Source: three-view drawing plus pictorial views. Frame: mm from the lowest corner of the part. Give positions to 0.01 mm unless a question says otherwise; leave off trailing zeros. Loops run counter-clockwise (first coordinate to the right, second up) from the corner with the lowest first, then second, coordinate; pieces in that order, holes last.
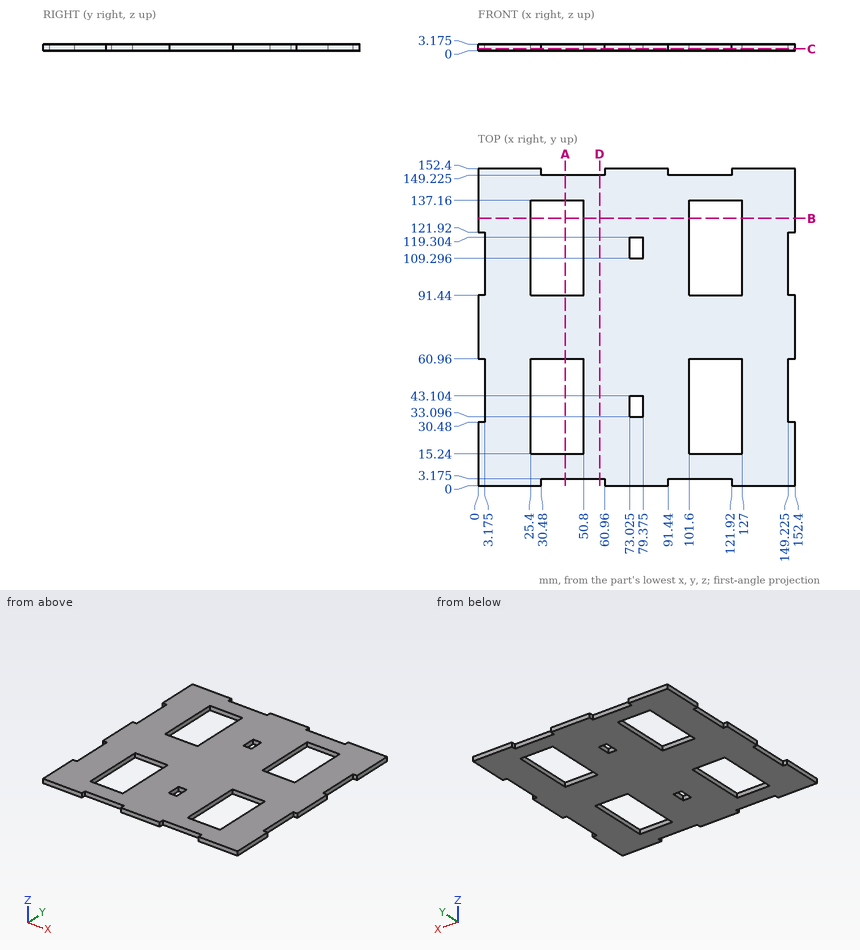
Q1. Section query A-A, the plane x = 42. Return loops of the section in (y, z) (3 decimals).
Q2. Material intervals for probe 1 along X at (y, z) = (114.5, 2.35) (3 decimals); probe 2 along X at (y, z) = (134.5, 1.65); probe 3 along Y at (x, z) = (116, 0.4) (3 decimals), sorted ascending.
Q3. Pin query (flat end, axial travel): pin 1 Ø1 at (x, z) = (75.5, 1.5) entering from -Y; pin 2 Ø1.6 at (y, z) = (113, 2) entering from +X (3 decimals); pin 3 Ø1.6 at (x, z) = (107.5, 1) entering from +Y (3 decimals); pin 4 Ø1 at (x, z) = (109, 1.5) entering from -Y (3 decimals). Return the tip coordinate at first contact, or that it passes through.
Q4. Section query B-B, the plane y = 128.5. Return loops of the section in (x, z) (3 decimals).
Q5. Section query D-D, the plane x = 58.5. Return loops of the section in (y, z) (3 decimals), and give its area (3 significant figures).
Q6. Section query C-C, the plane z = 0.8. State how many separate pieces and enclosed holes the cut face has, and give its area (3 significant figures).
Resolved:
1. outline: (3.175, 0) - (15.24, 0) - (15.24, 3.175) - (3.175, 3.175) - close; (60.96, 0) - (91.44, 0) - (91.44, 3.175) - (60.96, 3.175) - close; (137.16, 0) - (149.225, 0) - (149.225, 3.175) - (137.16, 3.175) - close
2. probe 1: x = 3.175 to 25.4, 50.8 to 73.025, 79.375 to 101.6, 127 to 149.225
2. probe 2: x = 0 to 25.4, 50.8 to 101.6, 127 to 152.4
2. probe 3: y = 3.175 to 15.24, 60.96 to 91.44, 137.16 to 149.225
3. pin 1: stops at y = 0
3. pin 2: stops at x = 149.225
3. pin 3: stops at y = 149.225
3. pin 4: stops at y = 3.175
4. outline: (0, 0) - (25.4, 0) - (25.4, 3.175) - (0, 3.175) - close; (50.8, 0) - (101.6, 0) - (101.6, 3.175) - (50.8, 3.175) - close; (127, 0) - (152.4, 0) - (152.4, 3.175) - (127, 3.175) - close
5. outline: (3.175, 0) - (149.225, 0) - (149.225, 3.175) - (3.175, 3.175) - close
5. area: 464 mm2
6. separate pieces: 1
6. enclosed holes: 6
6. area: 17,700 mm2
